CAD build for the part. Positions are in the model's coordinates, mm. A direction names the side the tool comes from. Coordinates: 2 decimals unless noted, no trailing zeros. Loops run counter-clockwise (first coordinate to the right, second up) from the corner with the lowest first, then second, coordinate; pieces in that order, holes last. Notation, with made-up numbers: (11, 33) -> (30, 33) arc R30 ccw to (30, 68) -> close; hole circle Ø4 at (-38.5, 7.25). An arc over 180 degrees is marked (long way). Write each question's results on one line, items separated by ' | '.
```python
from build123d import *

# Parameters (mm, degrees)
ESBO_O1_R                  = 7.5
RESSALTO_EXTRUS_O1_DEPTH   = 10
CORTE_EXTRUS_O1_DEPTH      = 15.577379737
CORTE_EXTRUS_O1_DEPTH_BACK = 15.577379737
ESBO_O2_W                  = 5
ESBO_O2_H                  = 15
CORTE_EXTRUS_O2_DEPTH      = 15.577379737
CORTE_EXTRUS_O2_DEPTH_BACK = 15.577379737
ESBO_O3_R                  = 2
CHANFRO1_SIZE              = 1
CHANFRO2_SIZE              = 1
CHANFRO3_SIZE              = 1


with BuildPart() as part:
    # Esboço1 → Ressalto-extrusão1 (new, symmetric)
    with BuildSketch(Plane(origin=(0, 0, 0), x_dir=(1, 0, 0), z_dir=(0, 1, 0))):
        with Locations(Location((0, 0, 0), (0, 0, 270))):
            Circle(ESBO_O1_R)
    extrude(amount=RESSALTO_EXTRUS_O1_DEPTH, both=True)

    # Esboço2 → Corte-extrusão1 (cut, two sides: drawn at the far end of the back side and taken through both)
    with BuildSketch(Plane(origin=(0, 0, 0), x_dir=(0, 0, -1), z_dir=(1, 0, 0)).offset(-CORTE_EXTRUS_O1_DEPTH_BACK)):
        with Locations((0, 2.5)):
            Rectangle(ESBO_O2_W, ESBO_O2_H)
    extrude(amount=CORTE_EXTRUS_O1_DEPTH + CORTE_EXTRUS_O1_DEPTH_BACK, mode=Mode.SUBTRACT)

    # Esboço3 → Corte-extrusão2 (cut, two sides: drawn at the far end of the back side and taken through both)
    with BuildSketch(Plane.XY.offset(-CORTE_EXTRUS_O2_DEPTH_BACK)):
        with Locations(Location((0, 5, 0), (0, 0, 90))):
            Circle(ESBO_O3_R)
    extrude(amount=CORTE_EXTRUS_O2_DEPTH + CORTE_EXTRUS_O2_DEPTH_BACK, mode=Mode.SUBTRACT)

    # Chanfro1
    chanfro1_edges = [part.edges().sort_by_distance(p)[0] for p in [
        (0, -10, -7.5),
    ]]
    chamfer(chanfro1_edges, length=CHANFRO1_SIZE)

    # Chanfro2
    chanfro2_edges = [part.edges().sort_by_distance(p)[0] for p in [
        (0, 10, -7.5),
        (-4.330127019, 10, 6.123724357),
        (0, 10, -2.5),
        (0, 10, 2.5),
    ]]
    chamfer(chanfro2_edges, length=CHANFRO2_SIZE)

    # Chanfro3
    chanfro3_edges = [part.edges().sort_by_distance(p)[0] for p in [
        (0, -5, -2.5),
        (0, -5, 2.5),
    ]]
    chamfer(chanfro3_edges, length=CHANFRO3_SIZE)


solid = part.part
```
Q1. Cut at A-A on x = 0. Write the cut outline in (y, z).
Results are:
outline: (-10, -6.5) -> (-9, -7.5) -> (3, -7.5) -> (3, -2.5) -> (-4, -2.5) -> (-5, -1.5) -> (-5, 1.5) -> (-4, 2.5) -> (3, 2.5) -> (3, 7.5) -> (-9, 7.5) -> (-10, 6.5) -> close; (7, -7.5) -> (9, -7.5) -> (10, -6.5) -> (10, -3.5) -> (9, -2.5) -> (7, -2.5) -> close; (7, 2.5) -> (9, 2.5) -> (10, 3.5) -> (10, 6.5) -> (9, 7.5) -> (7, 7.5) -> close
Q2. Which spindle directions (+Z, -Z, +X, -X, +Y, -Y) get a long thin tool onto all of the face, cutting with end or side? Do faces 5 (the cylindrical face through (0, 3, 5)), 6 (the flat face through (-0.1, 9.5, -3)). Say none if no direction does.
Results are:
face 5: +Z, -Z | face 6: +X, -X, +Y
Q3. Cut at B-B on y = 6.25. Write the cut outline in (x, z), and give its area (3 significant figures).
Results are:
outline: (-7.07, -2.5) arc R7.5 ccw to (-1.56, -7.34) -> (-1.56, -2.5) -> close; (-7.07, 2.5) -> (-1.56, 2.5) -> (-1.56, 7.34) arc R7.5 ccw to start; (1.56, -7.34) arc R7.5 ccw to (7.07, -2.5) -> (1.56, -2.5) -> close; (1.56, 2.5) -> (7.07, 2.5) arc R7.5 ccw to (1.56, 7.34) -> close | area: 72.2 mm^2
Q4. Drop flat-ended pins along their axis: pin 1 (6 mm diameter, centred on x = -4, y = -3.5, fed in from +Z); pin 2 (1 mm diameter, centred on y = -2.5, z = -6, fed in from -X); pin 3 (1.5 mm diameter, centred on x = -2.5, z = 0, fed in from +Y). Give the stop position or say it passes through.
Results are:
pin 1: z = 7.43 | pin 2: x = -5.1 | pin 3: y = -5
Q5. Wall check: L1, parallel to Y at x = 0, z = 5.4; L2, parallel to Y at x = 2.5, z = 0.25; L3, parallel to X at y = 5, z = 5.6. Give the ranges that are in metal, low to high. Write a range as from..to.
Results are:
L1: -10..3, 7..10 | L2: -10..-5 | L3: -4.99..-2, 2..4.99
Q6. Pull direction Z, two halves, no side cores. Call faces 1 (the conical face through (0.1, 9.8, -6.7)), 2 (the cylindrical face through (0.766, 6.847, -5.035)), 3 (the flat face through (-0.1, -4.5, -2)), 4 (the flat face through (-0.1, 9.5, 3)): +Z half, -Z half, draft (parallel to the pull), parting line (faces both ways), or undercut.
Results are:
face 1: -Z half | face 2: draft | face 3: undercut | face 4: undercut
Q7. Cut at C-C on y = -3.75. Write the cut outline in (x, z), and give its area (3 significant figures).
Results are:
outline: (-7.07, -2.5) arc R7.5 ccw to (7.07, -2.5) -> close; (-7.07, 2.5) -> (7.07, 2.5) arc R7.5 ccw to start | area: 103 mm^2
